Autodesk Inventor part; units mm, degrees
ref_plane "Work Plane1" through (-24, 0, -39) normal (0, 0, 1) x (1, 0, 0)
ref_plane "YZ Plane" through (0, 0, 0) normal (1, 0, 0) x (0, 1, 0)
ref_plane "XZ Plane" through (0, 0, 0) normal (0, 1, 0) x (-1, 0, 0)
sketch "Sketch1" plane through (0, 0, 0) normal (0, 1, 0) x (-1, 0, 0)
  line L0 (0, 0) -> (24, 0)
  line L1 (24, 0) -> (24, -78)
  line L2 (24, -78) -> (0, -78)
  line L3 (0, -78) -> (0, 0)
  dimension "d0" = 78
  dimension "d1" = 24
extrude "Extrusion1" add sketch "Sketch1" along normal blind 1.5
sketch "Sketch2" plane through (-24, 0, 0) normal (0, 0, 1) x (1, 0, 0)
  line L0 (24, 0) -> (0, 0)
  line L1 (0, 0) -> (24, 0)
  line L2 (24, 0) -> (24, 12)
  line L3 (24, 12) -> (0, 12)
  line L4 (0, 12) -> (0, 0)
  line L5 (24, 0) -> (24, 1.5)
  dimension "d4" = 12
extrude "Extrusion2" add sketch "Sketch2" against normal blind 18
sketch "Sketch3" plane through (0, 0, 0) normal (0, -1, 0) x (1, 0, 0)
  line L0 (-2, -10) -> (-22, -10)
  line L1 (-22, -10) -> (-22, -16)
  line L2 (-22, -16) -> (-2, -16)
  line L3 (-2, -16) -> (-2, -10)
  line L4 (-24, 0) -> (0, 0)
  line L5 (-24, -78) -> (-24, 0)
  line L6 (-2, -13) -> (-22, -13) construction
  line L7 (-12, 0) -> (-12, -78) construction
  line L8 (0, -78) -> (-24, -78) construction
  point P0 (-12, -13)
  dimension "d7" = 20
  dimension "d8" = 6
  dimension "d9" = 16
revolve "Revolution1" cut sketch "Sketch3" angle 360 about axis through (-2, 0, -10) along (-1, 0, 0)
ref_plane "Work Plane1" through (-24, 0, -39) normal (0, 0, 1) x (1, 0, 0)
sketch "Sketch4" plane through (0, 0, 0) normal (0, -1, 0) x (1, 0, 0)
  line L0 (0, 0) -> (0, -78) construction
  line L1 (0, -39) -> (-24, -39) construction
  line L2 (-24, -78) -> (-24, -18) construction
  line L3 (-24, -48.65) -> (0, -48.65)
  line L4 (0, -48.65) -> (0, -29.35)
  line L5 (0, -29.35) -> (-24, -29.35)
  line L6 (-24, -29.35) -> (-24, -48.65)
  line L7 (-24, -48.65) -> (0, -29.35) construction
  line L8 (0, -48.65) -> (-24, -29.35) construction
  point P0 (-12, -39)
  dimension "d12" = 19.3
extrude "Extrusion3" cut sketch "Sketch4" against normal up to surface (1.5 mm away)
sketch "Sketch5" plane through (0, 0, 0) normal (1, 0, 0) x (0, 0, -1)
  line L0 (29.35, 0) -> (29.35, 1.5)
  line L1 (29.35, 0) -> (27.85, 0)
  line L2 (27.85, 0) -> (27.85, 10.5)
  line L3 (27.85, 10.5) -> (29.35, 10.5)
  line L4 (29.35, 10.5) -> (29.35, 0)
  line L5 (27.85, 10.5) -> (39, 10.5)
  line L6 (39, 10.5) -> (39, 12)
  line L7 (39, 12) -> (27.85, 12)
  line L8 (27.85, 12) -> (27.85, 10.5)
  point P0 (0, 0)
  point P1 (29.35, 10.5)
  dimension "d15" = 1.5
  dimension "d16" = 10.5
  dimension "d17" = 1.5
  dimension "d18" = 11.15
extrude "Extrusion4" add sketch "Sketch5" against normal up to surface (24 mm away)
sketch "Sketch6" plane through (0, 0, 0) normal (0, -1, 0) x (1, 0, 0)
  line L0 (-2, -16) -> (-22, -16) construction
  line L1 (-24, -29.35) -> (0, -29.35) construction
  line L2 (-2, -16) -> (-22, -16) construction
  line L3 (-22, -16) -> (-22, -29.35) construction
  line L4 (-22, -29.35) -> (-2, -29.35) construction
  line L5 (-2, -29.35) -> (-2, -16) construction
  line L6 (-22, -16) -> (-22, -4) construction
  line L7 (-2, -22.675) -> (-22, -22.675) construction
  line L8 (-17, -22.675) -> (-7, -22.675) construction
  point P0 (0, 0)
  point P1 (-12, -22.675)
  dimension "d21" = 10
hole "Hole1" at (-7, 0, -22.675) at (-17, 0, -22.675) direction (0, 1, 0) diameter 3 depth 1.5
mirror "Mirror1" about plane through (-24, 0, -39) normal (0, 0, 1) of "Extrusion2", "Revolution1", "Extrusion4", "Hole1"
sketch "Sketch7" plane through (0, 0, 0) normal (1, 0, 0) x (0, 0, -1)
  line L0 (16, 0) -> (4, 0)
  arc A0 (13.25, 0) -> (6.75, 0) centre (10, 0) ccw
  line L1 (48.65, 0) -> (78, 0)
  arc A1 (71.25, 0) -> (64.75, 0) centre (68, 0) ccw
  arc A2 (16, 0) -> (4, 0) centre (10, 0) ccw
  arc A3 (74, 0) -> (62, 0) centre (68, 0) ccw
  line L2 (6.75, 0) -> (13.25, 0)
  line L3 (64.75, 0) -> (71.25, 0)
  point P0 (0, 0)
  dimension "d29" = 3.25
extrude "Extrusion5" cut sketch "Sketch7" against normal up to surface (24 mm away) contours L0 A0 | A1 L1
equation "\"d1\" = slider_top_width"
equation "\"d2\" = slider_top_thickness"
equation "\"d4\" = slider_top_height"
equation "\"d5\" = 2 * bearing_dist - bearing_diameter"
equation "\"d7\" = bearing_length"
equation "\"d8\" = 0.5 * bearing_diameter"
equation "\"d13\" = 2 * bearing_dist - bearing_diameter"
equation "\"d21\" = screw_dist"
equation "\"d22\" = screw_diameter"
equation "\"d29\" = 0.5 * rod_free_tolerance + 0.5 * slider_rod_diameter"
equation "\"slider_top_width\" = 24"
equation "\"slider_top_height\" = 12"
equation "\"slider_top_thickness\" = 1.5"
equation "\"bearing_length\" = 20"
equation "\"bearing_diameter\" = 12"
equation "\"bearing_dist\" = 15"
equation "\"lead_screw_outer_diameter\" = 12"
equation "\"screw_dist\" = 10"
equation "\"screw_diameter\" = 3"
equation "\"slider_rod_diameter\" = 6"
equation "\"rod_free_tolerance\" = 0.5"
properties part number "carriage_slider_top"
Could you check a few things on this model? Use its own coordinates, in mm. A direction names the side the tool comes from. Give positions to 0.01 mm unless a question says otherwise; leave off trailing zeros. Order: outer loops, then holes, each group sorted by start corner. A loop starts at its lowest first (then second) coordinate and runs counter-clockwise, first axis right, second up.
Q1. Suppose I cut it at A-A, the plane x = -17. Write out the boundary of the cut face in (y, z) (3 decimals).
Q2. If I drill on line 1 along Z through (x, y) = (-3, 11.25); line 2 along Z through (x, y) = (-6, 7.75); line 3 along Z through (x, y) = (-21.25, 1), over which ranges is the centre line in solid material (lowest first)?
Q3. For faces 5 (the flat face through (-12, 10.5, -39)), 6 (the flat face through (-2, 4, -10)), 7 (the flat face through (-12, 7, -50.15)), which set-ups out of +Z, -Z, +X, -X, +Y, -Y let a thin tool reach every point of the face, with its end or its side?
Q4. I'm going to push flat-ended pins straight in: P1, Ø3, axis at x = -7.5, z = -53, coming from the +Y side; P2, Ø2.5, axis at x = -7, z = -55.325, coming from the -Y side. Where does each tip first touch, or does it pass through?
Q5. Suppose I cut it at D-D, the plane y = 5. Write out the boundary of the cut face in (x, z), and give its area (3 significant figures).
Q6. Suppose I cut it at C-C, the plane z = -10. Write out the boundary of the cut face in (x, y).
Q7. Suppose I cut it at B-B, the plane y = 8.25. Write out the boundary of the cut face in (x, z).
Q8. We'd pull the mould along X, two halves only. Please class faces 1 (the cylindrical face through (-12, 6, -10)), 2 (the flat face through (-24, 11, -38)), 3 (the flat face through (-22, 4, -10)), 4 (the flat face through (-12, 7, -27.85)): +X half, -X half, draft (parallel to the pull), parting line (faces both ways), or undercut.
Solution:
1. outline: (0, -78) - (12, -78) - (12, -60) - (1.5, -60) - (1.5, -56.825) - (0, -56.825) - (0, -62) arc R6 cw to (0, -74) - close; (0, -53.825) - (1.5, -53.825) - (1.5, -50.15) - (12, -50.15) - (12, -27.85) - (1.5, -27.85) - (1.5, -24.175) - (0, -24.175) - (0, -29.35) - (10.5, -29.35) - (10.5, -48.65) - (0, -48.65) - close; (0, -21.175) - (1.5, -21.175) - (1.5, -18) - (12, -18) - (12, 0) - (0, 0) - (0, -4) arc R6 cw to (0, -16) - close
2. line 1: z = -78 to -60, -50.15 to -27.85, -18 to 0
2. line 2: z = -78 to -60, -50.15 to -48.65, -29.35 to -27.85, -18 to 0
2. line 3: z = -78 to -73.92, -62.08 to -48.65, -29.35 to -15.92, -4.08 to 0
3. face 5: +X, -X, -Y
3. face 6: -Y
3. face 7: +X, -X, +Y
4. P1: stops at y = 1.5
4. P2: passes through
5. outline: (-24, -78) - (0, -78) - (0, -60) - (-24, -60) - close; (-24, -50.15) - (0, -50.15) - (0, -48.65) - (-24, -48.65) - close; (-24, -29.35) - (0, -29.35) - (0, -27.85) - (-24, -27.85) - close; (-24, -18) - (0, -18) - (0, 0) - (-24, 0) - close; hole (-22, -71.32) - (-2, -71.32) - (-2, -64.68) - (-22, -64.68) - close; hole (-22, -13.32) - (-2, -13.32) - (-2, -6.68) - (-22, -6.68) - close
5. area: 671 mm2
6. outline: (-24, 3.25) - (-22, 3.25) - (-22, 6) - (-2, 6) - (-2, 3.25) - (0, 3.25) - (0, 12) - (-24, 12) - close
7. outline: (-24, -78) - (0, -78) - (0, -60) - (-24, -60) - close; (-24, -50.15) - (0, -50.15) - (0, -48.65) - (-24, -48.65) - close; (-24, -29.35) - (0, -29.35) - (0, -27.85) - (-24, -27.85) - close; (-24, -18) - (0, -18) - (0, 0) - (-24, 0) - close
8. face 1: undercut
8. face 2: -X half
8. face 3: undercut
8. face 4: draft
